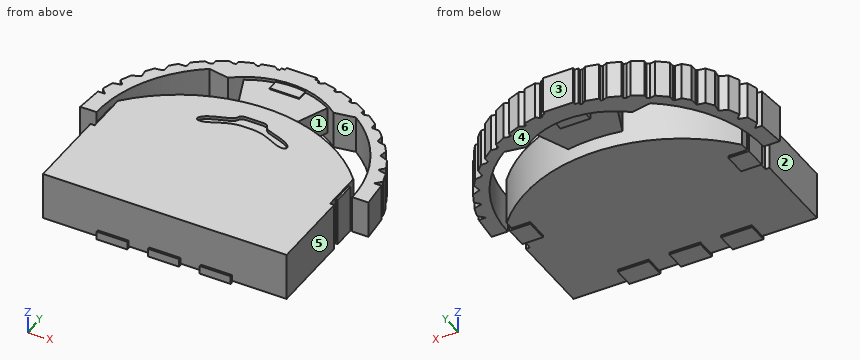
from build123d import *

# Parameters (mm, degrees)
SKETCH1_W            = 11.8
SKETCH1_H            = 4.1
BOSS_EXTRUDE1_DEPTH  = 2.3
SKETCH2_W            = 11.4
SKETCH2_H            = 2
BOSS_EXTRUDE2_DEPTH  = 2.3
BOSS_EXTRUDE3_START  = -0.1
SKETCH3_W            = 1
SKETCH3_H            = 1.1
BOSS_EXTRUDE3_DEPTH  = 2.3
BOSS_EXTRUDE4_START  = -0.1
SKETCH4_W            = 1.5
SKETCH4_H            = 1
BOSS_EXTRUDE4_DEPTH  = 0.4
LPATTERN1_COUNT      = 2
LPATTERN1_PITCH      = 2.5
LPATTERN1_COL_COUNT  = 2
LPATTERN1_COL_PITCH  = 2.5
BOSS_EXTRUDE5_DEPTH  = 2.3
CUT_EXTRUDE1_START   = 2.15
CUT_EXTRUDE1_DEPTH   = 0.15
BOSS_EXTRUDE6_START  = 0.1
SKETCH9_W            = 1.451153264
SKETCH9_H            = 0.139855477
SKETCH9_H_2          = 0.01502842
BOSS_EXTRUDE6_DEPTH  = 0.9
BOSS_EXTRUDE7_START  = 0.2
BOSS_EXTRUDE7_DEPTH  = 0.65
BOSS_EXTRUDE8_START  = 0.1
SKETCH12_W           = 1.44617415
SKETCH12_H           = 1.169902142
BOSS_EXTRUDE8_DEPTH  = 0.8
BOSS_EXTRUDE9_START  = 0.1
BOSS_EXTRUDE9_DEPTH  = 0.9
BOSS_EXTRUDE11_START = 0.1
BOSS_EXTRUDE11_DEPTH = 0.9


# Read off the part's stored shape, not the designer's step: Cut-Extrude1
with BuildPart() as part:
    # Sketch1 → Boss-Extrude1 (new body)
    with BuildSketch(Plane.XY):
        with Locations((5.9, 2.05)):
            Rectangle(SKETCH1_W, SKETCH1_H)
    extrude(amount=BOSS_EXTRUDE1_DEPTH)

    # Sketch2 → Boss-Extrude2 (add)
    with BuildSketch(Plane.XY):
        with Locations((5.903416876, 5.1)):
            Rectangle(SKETCH2_W, SKETCH2_H)
    extrude(amount=BOSS_EXTRUDE2_DEPTH)

    # Sketch3 → Boss-Extrude3 (add)
    with BuildSketch(Plane.XY.offset(BOSS_EXTRUDE3_START)):
        with Locations((0.601708438, 5.129355756)):
            Rectangle(SKETCH3_W, SKETCH3_H)
    boss_extrude3 = extrude(amount=BOSS_EXTRUDE3_DEPTH)

    # Mirror1: Boss-Extrude3 across plane
    add(boss_extrude3.mirror(Plane(origin=(5.9, 0, 0), x_dir=(0, 0, 1), z_dir=(1, 0, 0))))

    # Sketch4 → Boss-Extrude4 (add)
    with BuildSketch(Plane.XY.offset(BOSS_EXTRUDE4_START)):
        with Locations((5.898460375, 0.392479358)):
            Rectangle(SKETCH4_W, SKETCH4_H)
    boss_extrude4 = extrude(amount=BOSS_EXTRUDE4_DEPTH)

    # LPattern1: Boss-Extrude4 ×2
    with Locations(*[(i * LPATTERN1_PITCH, 0, 0) for i in range(1, LPATTERN1_COUNT)]):
        add(boss_extrude4)

    # LPattern1 col: Boss-Extrude4 ×2
    with Locations(*[(-i * LPATTERN1_COL_PITCH, 0, 0) for i in range(1, LPATTERN1_COL_COUNT)]):
        add(boss_extrude4)

    # Sketch7 → Boss-Extrude5 (add)
    with BuildSketch(Plane.XY):
        with BuildLine():
            Line((0.203416876, 6.1), (11.603416876, 6.1))
            ThreePointArc((11.603416876, 6.1), (5.903416876, 8.699567422), (0.203416876, 6.1))
        make_face()
    extrude(amount=BOSS_EXTRUDE5_DEPTH)

    # Cut-Extrude1 outline → Cut-Extrude1 (cut)
    with BuildSketch(Plane.XY.offset(CUT_EXTRUDE1_START)):
        with BuildLine():
            Line((5.9, 7.095183964), (5.9, 7.724501792))
            add(Edge.make_bspline(
                [(5.9, 7.724501792), (4.326937108, 7.822520939), (5.9, 7.319656572), (5.448711465, 7.255186781), (4.069057945, 7.229398865), (3.669345243, 7.087565325), (3.869201594, 7.158482095), (2.225221932, 6.120518466), (4.455876689, 6.146306382), (3.954545764, 6.281675552), (4.752437726, 7.113353242), (4.855589391, 7.061777409), (5.620353503, 7.110533179), (5.9, 7.095183964)],
                knots=[0, 0, 0, 0, 0, 0, 0, 0, 0, 0, 0, 0, 0, 0, 1, 1, 1, 1, 1, 1, 1, 1, 1, 1, 1, 1, 1, 1], degree=13))
        make_face()
    cut_extrude1 = extrude(amount=CUT_EXTRUDE1_DEPTH, mode=Mode.SUBTRACT)

    # Mirror2: Cut-Extrude1 across plane
    add(cut_extrude1.mirror(Plane(origin=(5.9, 0, 0), x_dir=(0, 0, 1), z_dir=(1, 0, 0))), mode=Mode.SUBTRACT)



with BuildPart() as body_2:
    # Sketch9 → Boss-Extrude6 (new, symmetric)
    with BuildSketch(Plane.XY.offset(1.15).offset(BOSS_EXTRUDE6_START)):
        with BuildLine():
            Line((2.355610817, 10.163701862), (3.34041857, 9.990053684))
            ThreePointArc((3.34041857, 9.990053684), (5.898836859, 10.90755899), (8.459580179, 9.996562953))
            Line((8.459580179, 9.996562953), (9.445513537, 10.163701862))
            ThreePointArc((9.445513537, 10.163701862), (5.900562177, 11.27807609), (2.355610817, 10.163701862))
        make_face()
        with BuildLine():
            ThreePointArc((-0.294894362, 5.129355756), (0.418313853, 7.968760684), (2.355610817, 10.163701862))
            ThreePointArc((2.355610817, 10.163701862), (5.900562177, 11.27807609), (9.445513537, 10.163701862))
            ThreePointArc((9.445513537, 10.163701862), (11.3828105, 7.968760684), (12.096018715, 5.129355756))
            Line((12.096018715, 5.129355756), (12.600483369, 5.129355756))
            ThreePointArc((12.600483369, 5.129355756), (10.879374358, 9.395993369), (6.813193458, 11.548337589))
            Line((6.813193458, 11.548337589), (6.625730117, 11.548337589))
            Line((6.625730117, 11.548337589), (6.625730117, 11.533309169))
            Line((6.625730117, 11.533309169), (5.174576853, 11.533309169))
            Line((5.174576853, 11.533309169), (5.174576853, 11.548337589))
            Line((5.174576853, 11.548337589), (4.987930896, 11.548337589))
            ThreePointArc((4.987930896, 11.548337589), (0.921749996, 9.395993369), (-0.799359016, 5.129355756))
            Line((-0.799359016, 5.129355756), (-0.294894362, 5.129355756))
        make_face()
        with Locations((5.900153485, 11.743092386)):
            Rectangle(SKETCH9_W, SKETCH9_H)
        with BuildLine():
            Line((5.174576853, 11.673164647), (5.174576853, 11.571323885))
            ThreePointArc((5.174576853, 11.571323885), (5.90015107, 11.610751105), (6.625730117, 11.571412879))
            Line((6.625730117, 11.571412879), (6.625730117, 11.673164647))
            Line((6.625730117, 11.673164647), (5.174576853, 11.673164647))
        make_face()
        with BuildLine():
            ThreePointArc((6.625730117, 11.571412879), (6.719543062, 11.560535503), (6.813193458, 11.548337589))
            Line((6.813193458, 11.548337589), (6.813193458, 11.673164647))
            Line((6.813193458, 11.673164647), (6.625730117, 11.673164647))
            Line((6.625730117, 11.673164647), (6.625730117, 11.571412879))
        make_face()
        with BuildLine():
            Line((4.987930896, 11.673164647), (4.987930896, 11.548337589))
            ThreePointArc((4.987930896, 11.548337589), (5.081173266, 11.560485266), (5.174576853, 11.571323885))
            Line((5.174576853, 11.571323885), (5.174576853, 11.673164647))
            Line((5.174576853, 11.673164647), (4.987930896, 11.673164647))
        make_face()
        with BuildLine():
            Line((5.174576853, 11.571323885), (5.174576853, 11.548337589))
            Line((5.174576853, 11.548337589), (6.625730117, 11.548337589))
            Line((6.625730117, 11.548337589), (6.625730117, 11.571412879))
            ThreePointArc((6.625730117, 11.571412879), (5.90015107, 11.610751105), (5.174576853, 11.571323885))
        make_face()
        with BuildLine():
            ThreePointArc((5.174576853, 11.571323885), (5.081173266, 11.560485266), (4.987930896, 11.548337589))
            Line((4.987930896, 11.548337589), (5.174576853, 11.548337589))
            Line((5.174576853, 11.548337589), (5.174576853, 11.571323885))
        make_face()
        with Locations((5.900153485, 11.540823379)):
            Rectangle(SKETCH9_W, SKETCH9_H_2)
        with BuildLine():
            Line((6.625730117, 11.548337589), (6.813193458, 11.548337589))
            ThreePointArc((6.813193458, 11.548337589), (6.719543062, 11.560535503), (6.625730117, 11.571412879))
            Line((6.625730117, 11.571412879), (6.625730117, 11.548337589))
        make_face()
    extrude(amount=BOSS_EXTRUDE6_DEPTH, both=True)



with BuildPart() as body_3:
    # Sketch11 → Boss-Extrude7 (new, symmetric)
    with BuildSketch(Plane.XY.offset(1.15).offset(BOSS_EXTRUDE7_START)):
        Polygon((8.224851185, 10.954397565), (5.972117123, 10.954397565), (3.66431816, 10.954397565), (4.823471696, 8.00789138), (5.903471696, 8.00789138), (6.988471696, 8.00789138), align=None)
    extrude(amount=BOSS_EXTRUDE7_DEPTH, both=True)


with BuildPart() as body_2_1:
    add(body_2.part)

    add(body_3.part)  # Boss-Extrude8 merges body 3
    # Sketch12 → Boss-Extrude8 (add, symmetric)
    with BuildSketch(Plane.XY.offset(1.15).offset(BOSS_EXTRUDE8_START)):
        with Locations((5.898836859, 10.90755899)):
            Rectangle(SKETCH12_W, SKETCH12_H)
    extrude(amount=BOSS_EXTRUDE8_DEPTH, both=True)

    # Sketch13 → Boss-Extrude9 (add, symmetric)
    with BuildSketch(Plane.XY.offset(1.15).offset(BOSS_EXTRUDE9_START)):
        Polygon((-1.08075819, 5.129355756), (-0.799359016, 5.129355756), (-0.671141909, 6.202084295), (-0.605509207, 6.451748475), (-0.958965207, 6.451748475), align=None)
    boss_extrude9 = extrude(amount=BOSS_EXTRUDE9_DEPTH, both=True)

    # Mirror3: Boss-Extrude9 across plane
    add(boss_extrude9.mirror(Plane(origin=(5.9, 0, 0), x_dir=(0, 0, 1), z_dir=(1, 0, 0))))


with BuildPart() as part_1:
    add(part.part)

    add(body_2_1.part)  # Boss-Extrude11 merges body 2
    # Sketch14 → Boss-Extrude11 (add, symmetric)
    with BuildSketch(Plane.XY.offset(1.15).offset(BOSS_EXTRUDE11_START)):
        Polygon((4.09350701, 11.514168222), (4.693813808, 11.65328598), (4.987930896, 11.450470962), (4.09350701, 11.286137141), align=None)
        Polygon((3.172552888, 11.201783695), (3.777829994, 11.433223707), (4.09350701, 11.286137141), (3.172552888, 10.950622256), align=None)
        Polygon((2.313751368, 10.77100106), (2.820138748, 11.052647163), (3.172552888, 10.950622256), (2.313751368, 10.477435247), align=None)
        Polygon((1.417632483, 10.151446182), (1.92347576, 10.542406597), (2.313751368, 10.477435247), (1.417632483, 9.837098648), align=None)
        Polygon((0.730905136, 9.506715824), (1.038871241, 9.827727461), (1.417632483, 9.837098648), (0.723421169, 9.107663948), align=None)
        Polygon((0.061798131, 8.677620181), (0.323212614, 9.049883319), (0.723421169, 9.107663948), (0.116840619, 8.296376932), align=None)
        Polygon((-0.534407657, 7.623618076), (-0.292532583, 8.132380345), (0.116840619, 8.296376932), (-0.279961599, 7.369172018), align=None)
        Polygon((-0.279961599, 7.369172018), (-0.716747876, 7.268090769), (-0.884396434, 6.725317521), (-0.622667426, 6.451748475), align=None)
    boss_extrude11 = extrude(amount=BOSS_EXTRUDE11_DEPTH, both=True)

    # Mirror4: Boss-Extrude11 across plane
    add(boss_extrude11.mirror(Plane(origin=(5.9, 0, 0), x_dir=(0, 0, 1), z_dir=(1, 0, 0))))


solid = part_1.part
Verification items for the finished model (mm, model axes). Face numbers are marked on the shaded views. A direction names the side the tool comes from. Give positions to 0.01 mm unless a question says otherwise; leave off trailing zeros. Write each loop counter-clockwise with the first axis right and the second up, starting at its lowest first coordinate (ties: lowest second). Pieces come first, ordered by that corner, then holes. Notation, with made-up numbers: M 8.5,-27.75 L 43.5,-27.75 A21 ccw 43.5,-23.75 Z; hole C 44.25,22 d7. An arc over 180 degrees is marked long. Put each result on its own line as item: value. Start each with the question number.
1. Scan lines: line 1 along Y through (x, z) = (5.25, 1.6); line 2 along X through (y, z) = (9.75, 1.1); line 3 along X through (y, z) = (6, 1.65). Record each from-to range of solid material in increasing order. Write a range as [from, to].
2. Draft check along Y on the marked faces 1, 2 and 3. Enter one of: +Y half, -Y half, draft (parallel to the pull), parting line (faces both ways), or undercut.
3. Section check B-B (y = 1.75). Record the cut outline in (x, z).
4. Set-up check for the marked faces 4, 5 and 6: record each of +Z, -Z, +X, -X, +Y, -Y from which the full face is reachable in a straight line by a thin tool's end or side.
5. Go/stop test with flat-tipped pins: pin 1 Ø4 at (x, y) = (7.5, 3) entering from -Z; pin 2 Ø0.6 at (x, y) = (7, 7) entering from +Z; pin 3 Ø0.8 at (x, z) = (11, 1) entering from -Y. Record where each tip stops, or that it passes through.
6. Section check A-A (z = 0.15). Record the cut outline in (x, y).
Answer list:
1. line 1: [0, 11.81]
1. line 2: [0.96, 1.83], [4.14, 7.72], [9.97, 10.84]
1. line 3: [-1, -0.23], [0.2, 11.6], [12.03, 12.8]
2. face 1: undercut
2. face 2: draft
2. face 3: +Y half
3. outline: M 0,0 L 11.8,0 L 11.8,2.3 L 0,2.3 Z
4. face 4: -Z, +Y
4. face 5: +Z, -Z, +X, -Y
4. face 6: +Z, -Z
5. pin 1: z = 0
5. pin 2: z = 2.3
5. pin 3: y = 0
6. outline: M 0,0 L 2.65,0 L 2.65,-0.11 L 4.15,-0.11 L 4.15,0 L 5.15,0 L 5.15,-0.11 L 6.65,-0.11 L 6.65,0 L 7.65,0 L 7.65,-0.11 L 9.15,-0.11 L 9.15,0 L 11.8,0 L 11.8,4.1 L 11.6,4.1 L 11.6,4.58 L 11.7,4.58 L 11.7,5.68 L 11.6,5.68 L 11.6,6.1 A7.55 ccw 0.2,6.1 L 0.2,5.68 L 0.1,5.68 L 0.1,4.58 L 0.2,4.58 L 0.2,4.1 L 0,4.1 Z
